For this review, take the finished solid that the model builds, in its own axes (mm). A direction names the side the tool comes from. Give positions to 0.01 mm unless a question says otherwise; leave off trailing zeros. Order: outer loops, then holes, each group sorted by start corner. A loop starts at its lowest first (then second) coordinate and runs counter-clockwise, first axis right, second up. Notation, with made-up numbers: M 1.5,17.5 L 46.5,17.5 A12 ccw 46.5,35.5 Z; hole C -11,-2.5 d1. An arc over 180 degrees is marked long. Answer as CSV lines item,"result". Start each with the question number.
1. Clearance check with flat-ended pins moving along their axes: P1, Ø6, axis at x = -11, y = -15.5, coming from the -Z side; P2, Ø11, axis at x = -8.5, y = -6.5, coming from the -Z side; P3, Ø3, axis at x = 12.5, y = -8.5, coming from the -Z side. State where each tip first meets the part, or that it passes through.
2. Machinability: for faces 4 (the cylindrical face through (-4.68, -12.52, 4.29)), 5 (the flat face through (10, -6, -3.175)), which of the approach directions +Z, -Z, +X, -X, +Y, -Y give a long, thin tool a straight path to every point of the face, cutting with its end or side? Answer none if there is none.
3. We need section A-A, the plane x = 0. Give the boundary of the cut face in (y, z) (3 decimals), and give its area (3 significant figures).
4. We need section D-D, the plane y = -23. Give the boundary of the cut face in (x, z) (3 decimals), and give its area (3 significant figures).
5. Mouldability with a two-part tool opening along Z and no side actions: class faces 1 (the cylindrical face through (15.14, -12.52, 4.77)), 2 (the flat face through (7, -25.4, 0)), 3 (the flat face through (-10, -6, 3.175)) as pulls with the +Z half, pulls with the -Z half, needs draft (parallel to the pull), parting line crosses it, or undercut.
6. For line 1 along Z through (x, y) = (0, -15.25) (3 decimals); line 2 along X through (y, z) = (-11.75, 5); line 3 along Z through (x, y) = (7, -9.5) (3 decimals), list the stretches that pass through material, from the lowest coordinate up.
7. We need section B-B, the plane y = -1.75. Give the boundary of the cut face in (x, z) (3 decimals), and give its area (3 significant figures).
8. We need section C-C, the plane x = -10. Give the boundary of the cut face in (y, z) (3 decimals).
from build123d import *

# Parameters (mm, degrees)
F0_R     = 15.875
F0_R_2   = 6.35
F1_DEPTH = 25.4
F2_R     = 3.175
F3_DEPTH = 25.4
F5_DEPTH = 25.4
F6_DEPTH = 25.4


with BuildPart() as f1:
    # F0 (on Front) → F1 (new body)
    with BuildSketch(Plane.XZ):
        Circle(F0_R)
        Circle(F0_R_2, mode=Mode.SUBTRACT)
    extrude(amount=F1_DEPTH)

    # F2 (on Right) → F3 (cut)
    with BuildSketch(Plane.YZ):
        Circle(F2_R)
    extrude(amount=-F3_DEPTH, mode=Mode.SUBTRACT)

    # F4 (on Right) → F5 (cut)
    with BuildSketch(Plane.YZ):
        with BuildLine():
            Line((0, 3.175), (-12.31459, 3.175))
            ThreePointArc((-12.31459, 3.175), (-15.48959, 0), (-12.31459, -3.175))
            Line((-12.31459, -3.175), (0, -3.175))
            Line((0, -3.175), (0, 3.175))
        make_face()
    extrude(amount=F5_DEPTH, mode=Mode.SUBTRACT)

    # F4 (on Right) → F6 (cut)
    with BuildSketch(Plane.YZ):
        with BuildLine():
            Line((0, 3.175), (-12.31459, 3.175))
            ThreePointArc((-12.31459, 3.175), (-15.48959, 0), (-12.31459, -3.175))
            Line((-12.31459, -3.175), (0, -3.175))
            Line((0, -3.175), (0, 3.175))
        make_face()
    extrude(amount=-F6_DEPTH, mode=Mode.SUBTRACT)


solid = f1.part
Result set:
1,P1,"z = -13.71"
1,P2,"z = -15.59"
1,P3,"z = -11.45"
2,face 4,"+Y, -Y"
2,face 5,"+X, -X, +Y"
3,outline,"M -25.4,-15.875 L 0,-15.875 L 0,-6.35 L -25.4,-6.35 Z; M -25.4,6.35 L 0,6.35 L 0,15.875 L -25.4,15.875 Z"
3,area,"484 mm2"
4,outline,"C 0,0 d31.75; hole C 0,0 d12.7"
4,area,"665 mm2"
5,face 1,"parting line crosses it"
5,face 2,"needs draft"
5,face 3,"undercut"
6,line 1,"-15.875 to -6.35, 6.35 to 15.875"
6,line 2,"-15.07 to -3.91, 3.91 to 15.07"
6,line 3,"-14.248 to -3.175, 3.175 to 14.248"
7,outline,"M -15.554,-3.175 A15.875 ccw 15.554,-3.175 L 5.499,-3.175 A6.35 cw -5.499,-3.175 Z; M -15.554,3.175 L -5.499,3.175 A6.35 cw 5.499,3.175 L 15.554,3.175 A15.875 ccw Z"
7,area,"542 mm2"
8,outline,"M -25.4,-12.329 L 0,-12.329 L 0,-3.175 L -12.315,-3.175 A3.175 cw -12.315,3.175 L 0,3.175 L 0,12.329 L -25.4,12.329 Z"
